```python
from build123d import *

# Parameters (mm, degrees)
SKETCH1_W               = 101.6
SKETCH1_H               = 101.6
SKETCH1_R               = 4.1656
BOSS_EXTRUDE1_DEPTH     = 3.175
F_1_4_20_TAPPED_HOLE1_D = 5.1054


with BuildPart() as part:
    # Sketch1 → Boss-Extrude1 (new, symmetric)
    with BuildSketch(Plane.XY):
        Rectangle(SKETCH1_W, SKETCH1_H)
        with Locations((-19.05, 0)):
            Circle(SKETCH1_R, mode=Mode.SUBTRACT)
        with Locations((19.05, 0)):
            Circle(SKETCH1_R, mode=Mode.SUBTRACT)
    extrude(amount=BOSS_EXTRUDE1_DEPTH, both=True)

    # Sketch2 → Cut-Revolve1 (revolve, cut)
    with BuildSketch(Plane(origin=(0, 0, 0), x_dir=(1, 0, 0), z_dir=(0, 1, 0))):
        Polygon((-10.5283, -3.175), (-19.05, 6.628094456), (-19.05, -3.175), align=None)
    cut_revolve1 = revolve(axis=Axis((-19.05, 0, -6.628094456), (0, 0, 1)), mode=Mode.SUBTRACT)

    # Sketch-Pattern1: Cut-Revolve1 at 1 more place
    with Locations((38.1, 0, 0)):
        add(cut_revolve1, mode=Mode.SUBTRACT)

    # 1/4-20 Tapped Hole1 (through all)
    with Locations(Plane.XY.offset(3.175)):
        with Locations((3.9624, -39.6875), (3.9624, 39.6875)):
            Hole(F_1_4_20_TAPPED_HOLE1_D / 2)


solid = part.part
```
For this review, take the finished solid that the model builds, in its own axes (mm). Coordinates: 2 decimals unless noted, no trailing zeros. Loops run counter-clockwise (first coordinate to the right, second up) from the corner with the lowest first, then second, coordinate; pieces in that order, holes last. Notation, with made-up numbers: (-35.75, -39.75) - (8.25, -39.75) arc R17 ccw to (8.25, -13.75) - close; hole circle Ø10 at (-6, -14.75). An arc over 180 degrees is marked (long way). Use one line per item in the form item = value. Start each with the question number.
1) Draft analysis for pull direction X (two halves, no side actions). For faces 1 (the face through (-1, -50.8, 0)), 2 (the face through (-50.8, -1, 0)), 3 (the face through (-14.875, 1.315, -1.593)), state which applies: released by +X, released by -X, zero draft, split by the parting line, or undercut.
2) Take a section at B-B (y = 0). State the section outline as (x, z) points (3 decimals), plus the area to 3 significant figures.
3) Take a section at A-A (x = 19.05). State the section outline as (y, z) points (3 decimals).
4) Take a section at C-C (z = -0.5). State the section outline as (x, y) points.
5) To check wall thickness, follow probe 1 along Y at (x, z) = (19.05, -2.8); probe 2 along Y at (x, z) = (5, -0.25); probe 3 along X at (y, z) = (6.5, 3). State the ranges of each line that lie inside material, in increasing order. Write a range as from..to.
6) For pin 1 (6.5 mm diameter, centred on x = 3.96, y = 39.69, fed in from +Z) (3 decimals), flat-tipped, find the tip position at first contact; note if it passes through.
From the geometry:
q1.face_1 = zero draft
q1.face_2 = released by -X
q1.face_3 = undercut
q2.outline = (-50.8, -3.175) - (-23.216, -3.175) - (-23.216, -1.836) - (-27.572, 3.175) - (-50.8, 3.175) - close; (-14.884, -3.175) - (14.884, -3.175) - (14.884, -1.836) - (10.528, 3.175) - (-10.528, 3.175) - (-14.884, -1.836) - close; (23.216, -3.175) - (50.8, -3.175) - (50.8, 3.175) - (27.572, 3.175) - (23.216, -1.836) - close
q2.area = 496 mm2
q3.outline = (-50.8, -3.175) - (-4.166, -3.175) - (-4.166, -1.836) - (-8.522, 3.175) - (-50.8, 3.175) - close; (4.166, -3.175) - (50.8, -3.175) - (50.8, 3.175) - (8.522, 3.175) - (4.166, -1.836) - close
q4.outline = (-50.8, -50.8) - (50.8, -50.8) - (50.8, 50.8) - (-50.8, 50.8) - close; hole circle Ø10.65 at (-19.05, 0); hole circle Ø5.11 at (3.96, -39.69); hole circle Ø5.11 at (3.96, 39.69); hole circle Ø10.65 at (19.05, 0)
q5.probe_1 = -50.8..-4.17, 4.17..50.8
q5.probe_2 = -50.8..-42.02, -37.36..37.36, 42.02..50.8
q5.probe_3 = -50.8..-24.32, -13.78..13.78, 24.32..50.8
q6.pin_1 = 3.175
